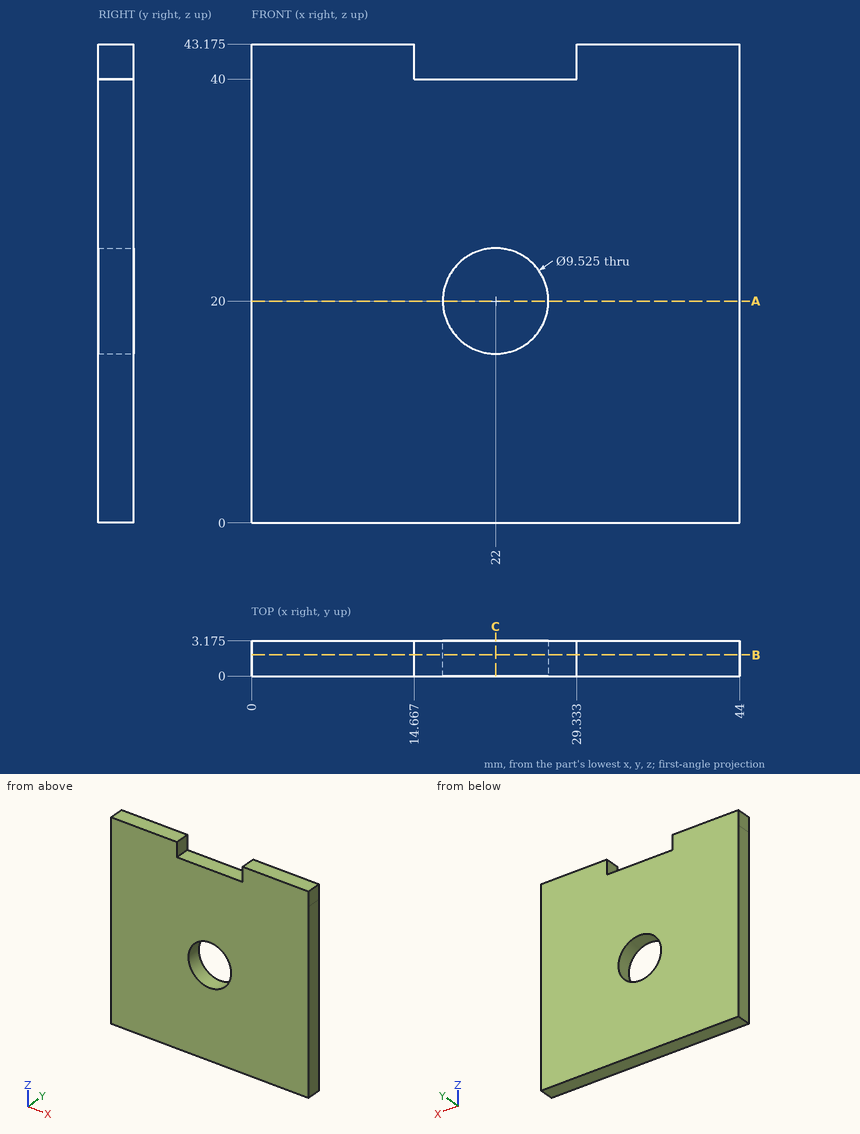
Drawing for the job (mm, zero at the part's lowest x, y, z). Round coordinates to 2 decimals unless told otherwise and drop trailing zeros. Write each loop counter-clockwise with the first axis right and the second up, starting at its lowest first coordinate (ties: lowest second). Pieces come first, ordered by that corner, then holes. Notation, with made-up numbers: M 61,40 L 94,40 A13 ccw 94,64 Z; hole C 12,22.5 d3. An arc over 180 degrees is marked long. Answer as a JSON object with one key per item and string values. Group by question number.
(1) Cut at A-A (z = 20). Give the cut face in (x, y) (1 decimal).
(2) Drill centre lines: L1, parallel to Z at x = 22, y = 1.6; L2, parallel to X at y = 0.25, z = 41; L3, parallel to Z at x = 28, y = 1.3. Where is each one in solid material? Low to high.
(3) Cut at B-B (y = 1.9). Give the cut face in (x, z) (1 decimal).
(4) Cut at C-C (x = 22). Give the cut face in (y, z) (1 decimal).
Responses:
{
 "1": {"outline": "M 0,0 L 17.2,0 L 17.2,3.2 L 0,3.2 Z; M 26.8,0 L 44,0 L 44,3.2 L 26.8,3.2 Z"},
 "2": {"L1": "z = 0 to 15.24, 24.76 to 40", "L2": "x = 0 to 14.67, 29.33 to 44", "L3": "z = 0 to 40"},
 "3": {"outline": "M 0,0 L 44,0 L 44,43.2 L 29.3,43.2 L 29.3,40 L 14.7,40 L 14.7,43.2 L 0,43.2 Z; hole C 22,20 d9.5"},
 "4": {"outline": "M 0,0 L 3.2,0 L 3.2,15.2 L 0,15.2 Z; M 0,24.8 L 3.2,24.8 L 3.2,40 L 0,40 Z"}
}
